```python
from build123d import *

# Parameters (mm, degrees)
F0_W     = 50.8
F0_H     = 25.4
F1_DEPTH = 3.175
F2_W     = 50.8
F2_H     = 19.05
F3_DEPTH = 3.175
F6_D     = 4.445
F8_D     = 4.445


with BuildPart() as f1:
    # F0 (on Top) → F1 (new body)
    with BuildSketch(Plane.XY):
        Rectangle(F0_W, F0_H)
    extrude(amount=F1_DEPTH)

    # F2 (on face) → F3 (join)
    with BuildSketch(Plane.XZ.offset(12.7)):
        with Locations((0, 9.525)):
            Rectangle(F2_W, F2_H)
    extrude(amount=F3_DEPTH)

    # F6 (through all)
    with Locations(Plane.XZ.offset(15.875)):
        with Locations((15.875, 12.7)):
            Hole(F6_D / 2)

    # F8 (through all)
    with Locations(Plane.XZ.offset(15.875)):
        with Locations((-15.875, 12.7)):
            Hole(F8_D / 2)


solid = f1.part
```
Geometry check sheet. Reference: the model listing, model coordinates, mm. A direction names the side the tool comes from. Coordinates: 2 decimals unless noted, no trailing zeros. Order: outer loops, then holes, each group sorted by start corner. A loop starts at its lowest first (then second) coordinate and runs counter-clockwise, first axis right, second up.
Q1. Draft check along X on faces 3 (the face through (0, -12.7, 11)), 4 (the face through (-17.995, -14.265, 13.368)), 5 (the face through (-25.4, -4, 3)), 6 (the face through (25.4, -4, 3)). Enter one of: released by +X, released by -X, zero draft, split by the parting line, or undercut.
Reply:
face 3: zero draft
face 4: undercut
face 5: released by -X
face 6: released by +X
Q2. Sectioned sample at A-A on z = 12.7. Record the cut outline in (x, y) (1 decimal).
Reply:
outline: (-25.4, -15.9) - (-18.1, -15.9) - (-18.1, -12.7) - (-25.4, -12.7) - close; (-13.7, -15.9) - (13.7, -15.9) - (13.7, -12.7) - (-13.7, -12.7) - close; (18.1, -15.9) - (25.4, -15.9) - (25.4, -12.7) - (18.1, -12.7) - close
Q3. Depth check by flat-ended pin: pin 1 Ø4 at (x, z) = (18.5, 15.5) entering from +Y; pin 2 Ø1 at (x, y) = (16, -6.5) entering from +Z (3 decimals); pin 3 Ø2.5 at (x, z) = (-15.875, 12.7) entering from +Y. Enter the tip coordinate at first touch or a pass-through.
Reply:
pin 1: stops at y = -12.7
pin 2: stops at z = 3.175
pin 3: passes through
Q4. Thickness scan on probe 1 along Y at (x, z) = (7, 14.5) (3 decimals); probe 2 along Z at (x, y) = (-9, 8.75) (3 decimals). Record the ranges inside material, lowest first.
Reply:
probe 1: y = -15.875 to -12.7
probe 2: z = 0 to 3.175
Q5. Tool access check on faces 1 (the face through (0, 12.7, 2)), 2 (the face through (0, 0, 3.175)). Record the directions out of +Z, -Z, +X, -X, +Y, -Y that give a thin tool (end or side, any length) a straight path to the whole face; none if there is none.
Reply:
face 1: +Z, -Z, +X, -X, +Y
face 2: +Z, +X, -X, +Y
Q6. Sectioned sample at D-D on z = 4.5. Record the cut outline in (x, y) (3 decimals), and give its area (3 significant figures).
Reply:
outline: (-25.4, -15.875) - (25.4, -15.875) - (25.4, -12.7) - (-25.4, -12.7) - close
area: 161 mm2
Q7. Sectioned sample at B-B on x = 17. Record the cut outline in (y, z) (3 decimals), and give its area (3 significant figures).
Reply:
outline: (-15.875, 0) - (12.7, 0) - (12.7, 3.175) - (-12.7, 3.175) - (-12.7, 10.783) - (-15.875, 10.783) - close; (-15.875, 14.617) - (-12.7, 14.617) - (-12.7, 19.05) - (-15.875, 19.05) - close
area: 129 mm2
Q8. Sectioned sample at C-C on y = 10.5. Record the cut outline in (x, z) (3 decimals).
Reply:
outline: (-25.4, 0) - (25.4, 0) - (25.4, 3.175) - (-25.4, 3.175) - close
